Part model, mm, in its own coordinate system. Face numbers are marked on the shaded views. A direction names the side the tool comes from. Give positions to 0.01 mm unless a question says otherwise; leave off trailing zeros. Order: outer loops, then holes, each group sorted by start corner. A loop starts at its lowest first (then second) coordinate and runs counter-clockwise, first axis right, second up. Notation, with made-up numbers: (1.5, 64) - (18.5, 64) arc R31 ccw to (18.5, 95) - close; hole circle Ø7 at (41, 10.25). An arc over 180 degrees is marked (long way). Use one line per item in the form item = value. Start each with the question number.
1. Pull direction Z, two halves, no side cores. Call the marked faces 1, 2, 3 and 4: +Z half, -Z half, draft (parallel to the pull), parting line (faces both ways), or undercut.
2. Tool access for the marked faces 5 and 6: list every direction of +Z, -Z, +X, -X, +Y, -Y with a clear straight run to the whole face (end or side of a thin tool).
3. Band-saw the part on D-D, the plane x = 53. List the corners of the cut face in (y, z), plus the area to 3 significant figures.
4. Band-saw the part on C-C, the plane y = 38.5. List the corners of the cut face in (x, z), plus the area to 3 significant figures.
5. Band-saw the part on B-B, the plane z = 55. List the corners of the cut face in (x, y), plus the area to 3 significant figures.
6. Drill centre lines: line 1 (Z direction, x = 0, y = 5); line 2 (Z direction, x = 64, y = 41.5); line 3 (X direction, y = 84, z = -35.5). Where is each one in solid material? Low to high.
7. Pin check, flat tip, straight feed: P1, Ø6, axis at x = -98, z = -45.5, coming from the +Y side. Stop position of the tip, or through.
8. Band-saw the part on A-A, the plane x = 0. List the corners of the cut face in (y, z), plus the area to 3 significant figures.
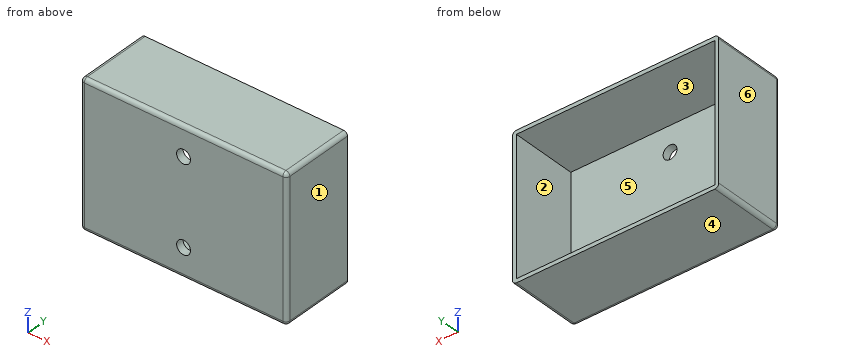
from build123d import *

# Parameters (mm, degrees)
SKETCH1_W           = 265
SKETCH1_H           = 185
BOSS_EXTRUDE1_DEPTH = 95
SKETCH2_W           = 255
SKETCH2_H           = 175
CUT_EXTRUDE1_DEPTH  = 85
CUT_EXTRUDE2_REACH  = 97
SKETCH6_R           = 8.89
FILLET1_R           = 5


with BuildPart() as part:
    # Sketch1 → Boss-Extrude1 (new body)
    with BuildSketch(Plane(origin=(0, 0, 0), x_dir=(1, 0, 0), z_dir=(0, 1, 0))):
        Rectangle(SKETCH1_W, SKETCH1_H)
    extrude(amount=BOSS_EXTRUDE1_DEPTH)

    # Sketch2 → Cut-Extrude1 (cut)
    with BuildSketch(Plane(origin=(0, 95, 0), x_dir=(1, 0, 0), z_dir=(0, 1, 0))):
        Rectangle(SKETCH2_W, SKETCH2_H)
    extrude(amount=-CUT_EXTRUDE1_DEPTH, mode=Mode.SUBTRACT)

    # Sketch6 → Cut-Extrude2 (cut, up to next)
    with BuildSketch(Plane.XZ, mode=Mode.PRIVATE) as cut_extrude2_sk1:
        with Locations((0, 55)):
            Circle(SKETCH6_R)
    cut_extrude2_tool1 = extrude(cut_extrude2_sk1.sketch, amount=-CUT_EXTRUDE2_REACH, mode=Mode.PRIVATE) & part.part
    add(cut_extrude2_tool1.solids().sort_by_distance((0, 0, 55))[0], mode=Mode.SUBTRACT)
    # Sketch6 → Cut-Extrude2 (cut, up to next)
    with BuildSketch(Plane.XZ, mode=Mode.PRIVATE) as cut_extrude2_sk2:
        with Locations((0, -55)):
            Circle(SKETCH6_R)
    cut_extrude2_tool2 = extrude(cut_extrude2_sk2.sketch, amount=-CUT_EXTRUDE2_REACH, mode=Mode.PRIVATE) & part.part
    add(cut_extrude2_tool2.solids().sort_by_distance((0, 0, -55))[0], mode=Mode.SUBTRACT)

    # Fillet1
    fillet1_edges = [part.edges().sort_by_distance(p)[0] for p in [
        (0, 0, 92.5),
        (-132.5, 0, 0),
        (0, 0, -92.5),
        (132.5, 0, 0),
        (132.5, 47.5, 92.5),
        (-132.5, 47.5, 92.5),
        (-132.5, 47.5, -92.5),
        (132.5, 47.5, -92.5),
    ]]
    fillet(fillet1_edges, radius=FILLET1_R)


solid = part.part
From the geometry:
q1.face_1 = draft
q1.face_2 = undercut
q1.face_3 = undercut
q1.face_4 = -Z half
q2.face_5 = +Y
q2.face_6 = +Z, -Z, -X, +Y, -Y
q3.outline = (0, -87.5) arc R5 ccw to (5, -92.5) - (95, -92.5) - (95, -87.5) - (10, -87.5) - (10, 87.5) - (95, 87.5) - (95, 92.5) - (5, 92.5) arc R5 ccw to (0, 87.5) - close
q3.area = 2,690 mm²
q4.outline = (-132.5, -87.5) arc R5 ccw to (-127.5, -92.5) - (127.5, -92.5) arc R5 ccw to (132.5, -87.5) - (132.5, 87.5) arc R5 ccw to (127.5, 92.5) - (-127.5, 92.5) arc R5 ccw to (-132.5, 87.5) - close; hole (-127.5, -87.5) - (127.5, -87.5) - (127.5, 87.5) - (-127.5, 87.5) - close
q4.area = 4,380 mm²
q5.outline = (-132.5, 5) arc R5 ccw to (-127.5, 0) - (-8.89, 0) - (-8.89, 10) - (-127.5, 10) - (-127.5, 95) - (-132.5, 95) - close; (8.89, 0) - (127.5, 0) arc R5 ccw to (132.5, 5) - (132.5, 95) - (127.5, 95) - (127.5, 10) - (8.89, 10) - close
q5.area = 3,310 mm²
q6.line_1 = -92.5 to -63.89, -46.11 to 46.11, 63.89 to 92.5
q6.line_2 = -92.5 to -87.5, 87.5 to 92.5
q6.line_3 = -132.5 to -127.5, 127.5 to 132.5
q7.P1 = 10
q8.outline = (0, -87.5) arc R5 ccw to (5, -92.5) - (95, -92.5) - (95, -87.5) - (10, -87.5) - (10, -63.89) - (0, -63.89) - close; (0, -46.11) - (10, -46.11) - (10, 46.11) - (0, 46.11) - close; (0, 63.89) - (10, 63.89) - (10, 87.5) - (95, 87.5) - (95, 92.5) - (5, 92.5) arc R5 ccw to (0, 87.5) - close
q8.area = 2,330 mm²
